Design review of the part shown in the three views and the two pictorial views. Dimensions are in mm from the part's minimum x, y and z. A direction names the side the tool comes from. Give positions to 0.01 mm unless a question says otherwise; leave off trailing zeros. Write each loop counter-clockwise with the first axis right and the second up, starting at its lowest first coordinate (ties: lowest second). Pieces come first, ordered by that corner, then holes. Notation, with made-up numbers: M -19,25 L 4,25 A8 ccw 4,35 Z; hole C -36.75,53 d3. An arc over 180 degrees is marked long. Write item = value, one per line.
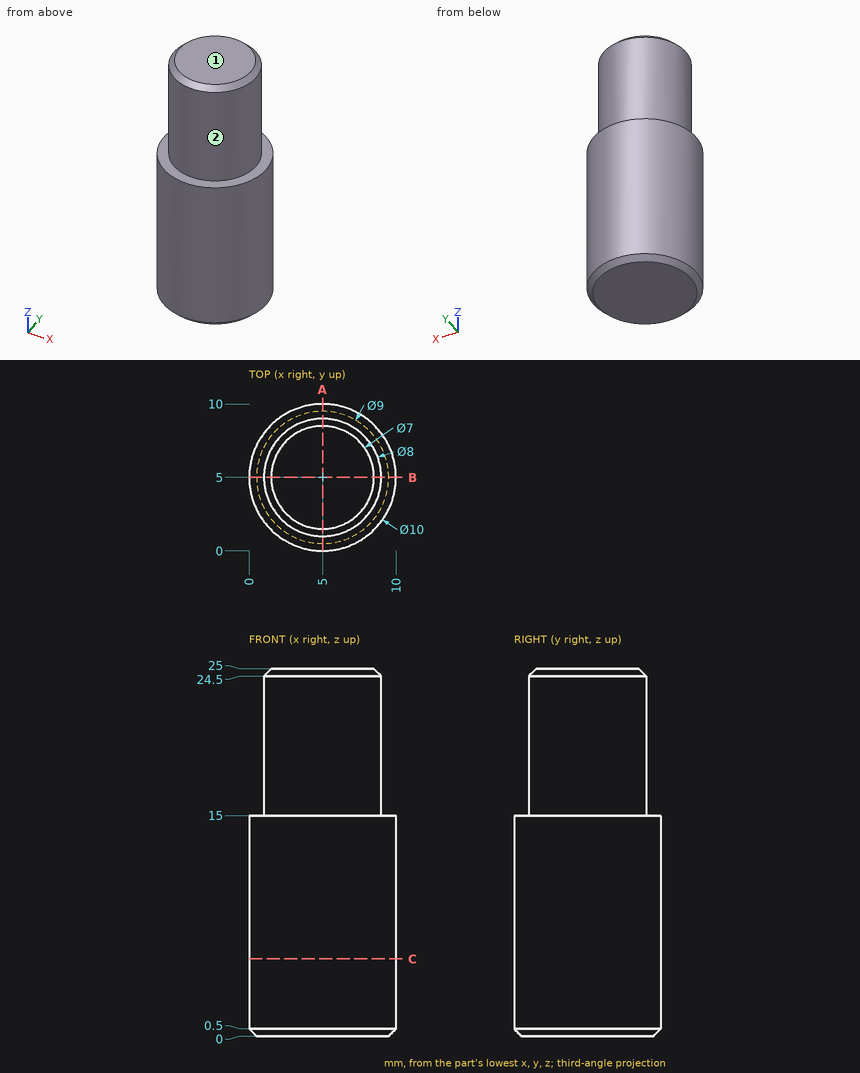
1. We need section C-C, the plane z = 5.25. Write out the cut boundary in (x, y).
Responses:
outline = C 5,5 d10
2. Insertion check: P1, Ø5, axis at y = 3.5, z = 20.5, coming from the +X side; P2, Ø3, axis at x = 3, y = 2, coming from the +Z side. Each pin has a flat end and moves straight along its axis. Give the tip position at first contact, or say it passes through.
Responses:
P1 = 9
P2 = 25
3. We need section A-A, the plane x = 5. Write out the cut boundary in (y, z).
Responses:
outline = M 0,0.5 L 0.5,0 L 9.5,0 L 10,0.5 L 10,15 L 9,15 L 9,24.5 L 8.5,25 L 1.5,25 L 1,24.5 L 1,15 L 0,15 Z
4. For line 1 along Y through (x, z) = (5.25, 6); line 2 along Y through (x, z) = (3.25, 21); line 3 along X through (y, z) = (6.75, 13), list the stretches that pass through material, from the lowest coordinate up. Write a range as from..to.
Responses:
line_1 = 0.01..9.99
line_2 = 1.4..8.6
line_3 = 0.32..9.68
5. Machinability: for the marked faces 1 and 2, which of the approach directions +Z, -Z, +X, -X, +Y, -Y give a long, thin tool a straight path to every point of the face, cutting with its end or side? Answer none if there is none.
Responses:
face_1 = +Z, +X, -X, +Y, -Y
face_2 = +Z
